Check sheet for the drawn part. Datum: minimum x, y, z corner. Units: mm. Coordinates: 2 decimals unless noted, no trailing zeros. Loops run counter-clockwise (first coordinate to the right, second up) from the corner with the lowest first, then second, coordinate; pieces in that order, holes last. Notation, with made-up numbers: (44, 16.25) - (57, 16.25) arc R22 ccw to (57, 52.25) - close; hole circle Ø1 at (81, 46.25). An arc over 180 degrees is marked (long way). Write item = value, one per line. Start each with the question number.
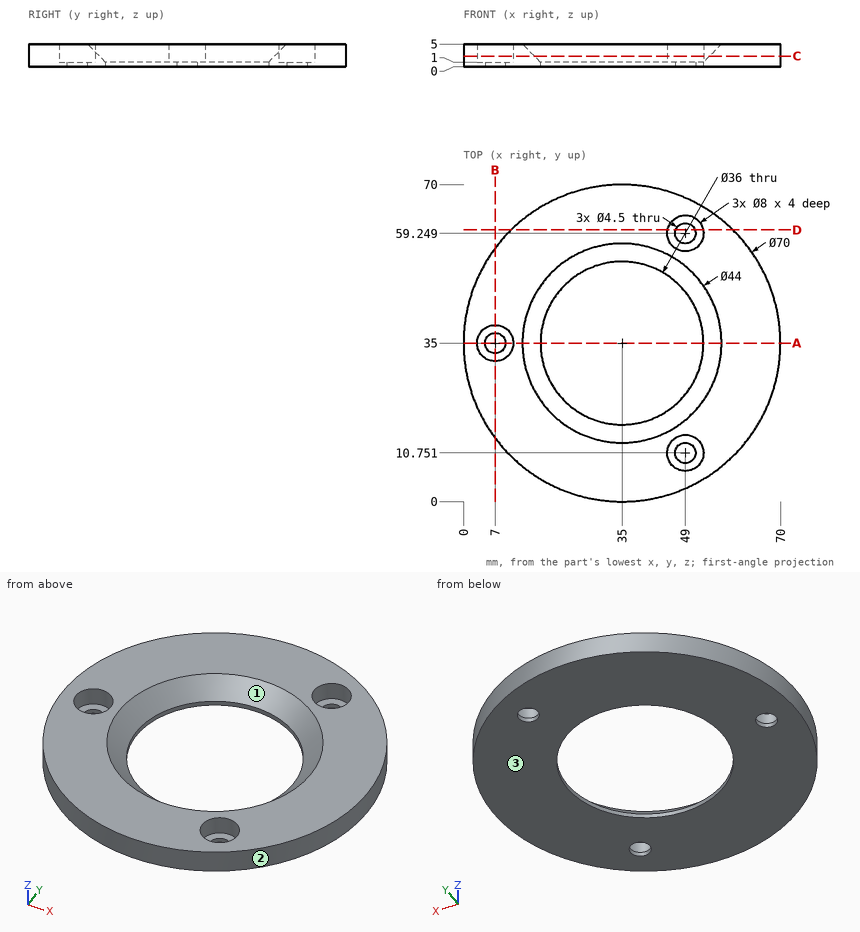
(1) Sectioned sample at A-A on y = 35. Enter the section's corners in (x, z).
(2) Sectioned sample at B-B on x = 7. Enter the section's corners in (y, z).
(3) Sectioned sample at D-D on y = 60. Enter the section's corners in (x, z) (1 decimal), plus the area to 3 significant figures.
(4) Scan lines: line 1 (Y direction, x = 49, z = 0.4) (1 decimal); line 2 (Y direction, x = 35, z = 0.35); line 3 (Y direction, x = 52, z = 3.05) (1 decimal). Record each from-to range of solid material in increasing order.
(5) Depth check by flat-ended pin: pin 1 (2.5 mm diameter, centred on x = 49, y = 10.75, fed in from +Z); pin 2 (4 mm diameter, centred on x = 7.5, y = 36.5, fed in from +Z); pin 3 (2 mm diameter, centred on x = 43.5, z = 1.5, fed in from +Y). Enter the tip coordinate at first touch or a pass-through.
(6) Draft check along X on the marked faces 1, 2 and 3. Enter one of: pulls with the +X half, pulls with the -X half, needs draft (parallel to the pull), parting line crosses it, or undercut.
(7) Sectioned sample at C-C on z = 2.35. Enter the section's corners in (x, y).
Working result:
q1.outline = (0, 0) - (4.75, 0) - (4.75, 1) - (3, 1) - (3, 5) - (0, 5) - close; (9.25, 0) - (17, 0) - (17, 1) - (13, 5) - (11, 5) - (11, 1) - (9.25, 1) - close; (53, 0) - (70, 0) - (70, 5) - (57, 5) - (53, 1) - close
q2.outline = (14, 0) - (32.75, 0) - (32.75, 1) - (31, 1) - (31, 5) - (14, 5) - close; (37.25, 0) - (56, 0) - (56, 5) - (39, 5) - (39, 1) - (37.25, 1) - close
q3.outline = (10.5, 0) - (46.9, 0) - (46.9, 1) - (45.1, 1) - (45.1, 5) - (10.5, 5) - close; (51.1, 0) - (59.5, 0) - (59.5, 5) - (52.9, 5) - (52.9, 1) - (51.1, 1) - close
q3.area = 209 mm2
q4.line_1 = 2.9 to 8.5, 13 to 23.7, 46.3 to 57, 61.5 to 67.1
q4.line_2 = 0 to 17, 53 to 70
q4.line_3 = 4.4 to 8.1, 13.4 to 24.4, 45.6 to 56.6, 61.9 to 65.6
q5.pin_1 = through
q5.pin_2 = 1
q5.pin_3 = 69.19
q6.face_1 = undercut
q6.face_2 = parting line crosses it
q6.face_3 = needs draft
q7.outline = circle Ø70 at (35, 35); hole circle Ø8 at (7, 35); hole circle Ø38.7 at (35, 35); hole circle Ø8 at (49, 10.75); hole circle Ø8 at (49, 59.25)
